Here's the drawing with two shaded views (mm, measured from the low corner). I have some questions. Give positions to 0.01 mm unless a question says otherwise; leave off trailing zeros. Write each loop counter-clockwise with the first axis right and the second up, starting at its lowest first coordinate (ties: lowest second). Pieces come first, ordered by that corner, then holes.
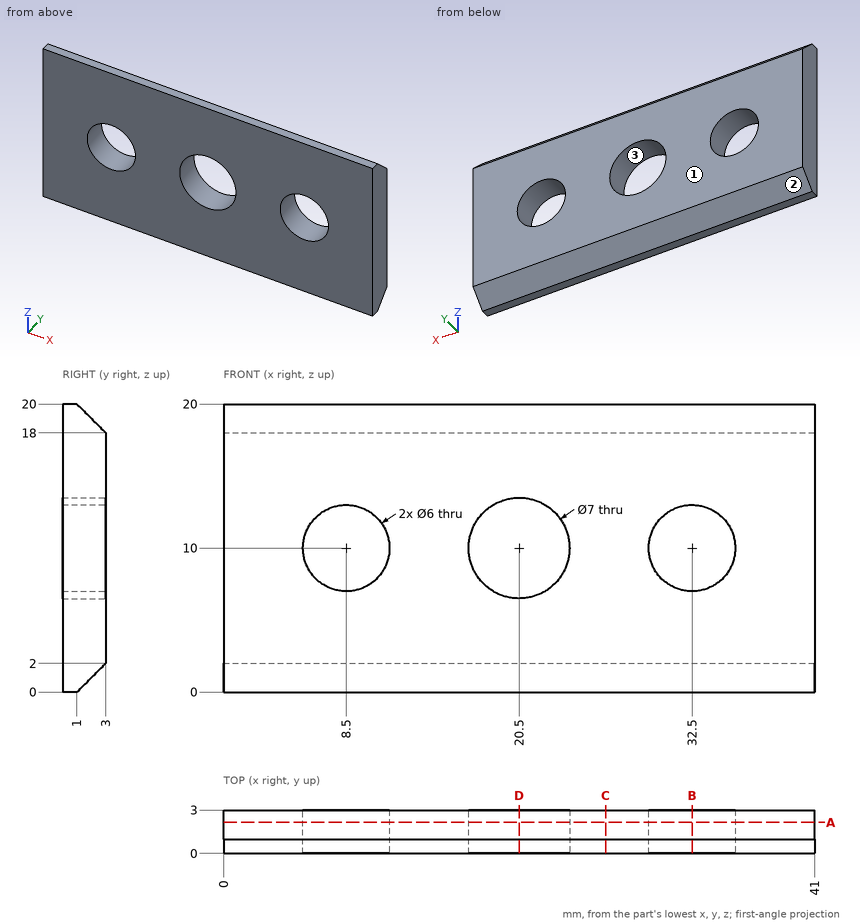
(1) Imagine slicing it at D-D, the plane x = 20.5. Write out the boundary of the cut face in (y, z), plus the area to 3 significant figures.
Returned:
outline: (0, 0) - (1, 0) - (3, 2) - (3, 6.5) - (0, 6.5) - close; (0, 13.5) - (3, 13.5) - (3, 18) - (1, 20) - (0, 20) - close
area: 35.0 mm2
(2) Imagine slicing it at C-C, the plane x = 26.5. Write out the boundary of the cut face in (y, z).
Returned:
outline: (0, 0) - (1, 0) - (3, 2) - (3, 18) - (1, 20) - (0, 20) - close
(3) If I drill on L1, parallel to X at y = 2.1, z = 10; L2, parallel to X at y = 2.75, z = 8; L3, parallel to Z at x = 31, y = 2.6, over which ranges is the centre line in solid material (lowest first)?
Returned:
L1: x = 0 to 5.5, 11.5 to 17, 24 to 29.5, 35.5 to 41
L2: x = 0 to 6.26, 10.74 to 17.63, 23.37 to 30.26, 34.74 to 41
L3: z = 1.6 to 7.4, 12.6 to 18.4
(4) Imagine slicing it at B-B, the plane x = 32.5. Write out the boundary of the cut face in (y, z), plus the area to 3 significant figures.
Returned:
outline: (0, 0) - (1, 0) - (3, 2) - (3, 7) - (0, 7) - close; (0, 13) - (3, 13) - (3, 18) - (1, 20) - (0, 20) - close
area: 38.0 mm2
(5) Imagine slicing it at A-A, the plane y = 2.15. Write out the boundary of the cut face in (x, z), plus the area to 3 significant figures.
Returned:
outline: (0, 1.15) - (41, 1.15) - (41, 18.85) - (0, 18.85) - close; hole circle Ø6 at (8.5, 10); hole circle Ø7 at (20.5, 10); hole circle Ø6 at (32.5, 10)
area: 631 mm2
(6) If we mould it in two halves opening along Z, with no side actions, what happens to the marked faces 1, 2 and 3? For each: +Z half, -Z half, draft (parallel to the pull), parting line (faces both ways), or undercut.
Returned:
face 1: draft
face 2: -Z half
face 3: undercut
(7) Will these pins go through, and if not, where does the flat tip stop? P1, Ø6.5, axis at x = 20.5, z = 10, coming from the -Y side; P2, Ø1, axis at x = 16, y = 2.5, coming from the -Z side.
Returned:
P1: passes through
P2: stops at z = 1
